```python
from build123d import *

# Parameters (mm, degrees)
F3_DEPTH = 15
F2_R     = 6.1
F4_DEPTH = 20
F5_R     = 3.25
F6_DEPTH = 20
F5_R_2   = 13.7
F7_DEPTH = 1.3
F2_R_2   = 20
F2_R_3   = 8.5
F8_DEPTH = 0.4


with BuildPart() as f1:
    # F0 (on Right) → F1 (revolve)
    with BuildSketch(Plane.YZ):
        with BuildLine():
            Line((0, 10), (0, 0))
            Line((0, 0), (15, 0))
            add(Edge.make_bspline(
                [(12.5, 17.5), (13.5772919142, 11.6888974623), (14.2886459571, 5.8444487312), (15, 0)],
                knots=[0.5019201889, 0.5019201889, 0.5019201889, 0.5019201889, 1, 1, 1, 1], degree=3))
            Line((12.5, 17.5), (8.4409715081, 17.5))
            ThreePointArc((8.4409715081, 17.5), (5.6457948953, 12.1458674864), (0, 10))
        make_face()
        with BuildLine():
            Line((8.4409715081, 17.5), (12.5, 17.5))
            add(Edge.make_bspline(
                [(8.5, 35), (9.9572008854, 29.1779541329), (11.4144017707, 23.3559082658), (12.5, 17.5)],
                knots=[0, 0, 0, 0, 0.5019201889, 0.5019201889, 0.5019201889, 0.5019201889], degree=3))
            Line((8.5, 35), (0, 35))
            Line((0, 35), (0, 27))
            ThreePointArc((0, 27), (6.0104076401, 24.5104076401), (8.5, 18.5))
            ThreePointArc((8.5, 18.5), (8.4852300446, 17.9991296668), (8.4409715081, 17.5))
        make_face()
    revolve(axis=Axis((0, 0, 17.5), (0, 0, -1)))

    # F0 (on Right) → F3 (cut, symmetric)
    with BuildSketch(Plane.YZ):
        with BuildLine():
            Line((0, 17.5), (0, 10))
            ThreePointArc((0, 10), (5.6457948953, 12.1458674864), (8.4409715081, 17.5))
            Line((8.4409715081, 17.5), (0, 17.5))
        make_face()
        with BuildLine():
            ThreePointArc((-8.4409715081, 17.5), (-5.6457948953, 12.1458674864), (0, 10))
            Line((0, 10), (0, 17.5))
            Line((0, 17.5), (-8.4409715081, 17.5))
        make_face()
        with BuildLine():
            ThreePointArc((0, 27), (-6.3541325136, 24.1457948953), (-8.4409715081, 17.5))
            Line((-8.4409715081, 17.5), (0, 17.5))
            Line((0, 17.5), (0, 27))
        make_face()
        with BuildLine():
            Line((0, 27), (0, 17.5))
            Line((0, 17.5), (8.4409715081, 17.5))
            ThreePointArc((8.4409715081, 17.5), (8.4852300446, 17.9991296668), (8.5, 18.5))
            ThreePointArc((8.5, 18.5), (6.0104076401, 24.5104076401), (0, 27))
        make_face()
    extrude(amount=F3_DEPTH, both=True, mode=Mode.SUBTRACT)

    # F2 (on face) → F4 (cut)
    with BuildSketch(Plane.XY.offset(35)):
        Circle(F2_R)
    extrude(amount=-F4_DEPTH, mode=Mode.SUBTRACT)

    # F5 (on face) → F6 (cut)
    with BuildSketch(Plane(origin=(0, 0, 0), x_dir=(1, 0, 0), z_dir=(0, 0, -1))):
        Circle(F5_R)
    extrude(amount=-F6_DEPTH, mode=Mode.SUBTRACT)

    # F5 (on face) → F7 (cut)
    with BuildSketch(Plane(origin=(0, 0, 0), x_dir=(1, 0, 0), z_dir=(0, 0, -1))):
        Circle(F5_R_2)
        Circle(F5_R, mode=Mode.SUBTRACT)
    extrude(amount=-F7_DEPTH, mode=Mode.SUBTRACT)

    # F2 (on face) → F8 (join)
    with BuildSketch(Plane.XY.offset(35)):
        Circle(F2_R_2)
        Circle(F2_R_3, mode=Mode.SUBTRACT)
        Circle(F2_R_3)
        Circle(F2_R, mode=Mode.SUBTRACT)
    extrude(amount=F8_DEPTH)


solid = f1.part
```
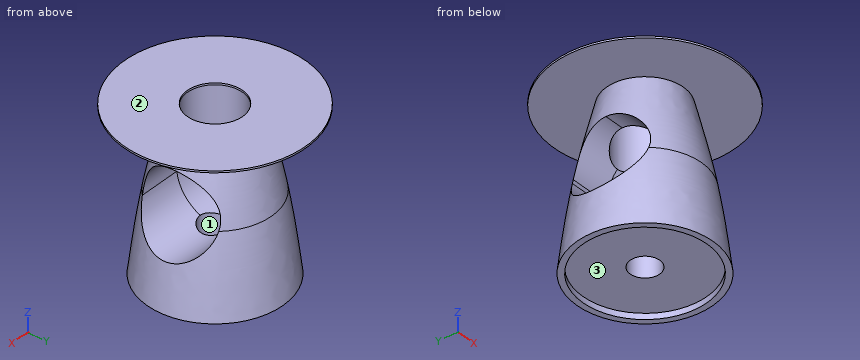
For this review, take the finished solid that the model builds, in its own axes (mm). Face numbers are marked on the shaded views. Round coordinates to 2 decimals unless told otherwise and drop trailing zeros.
Q1. Add section A-A on y = -4.5. Give the number of separate pieces and of enclosed holes in the cut face, plus the area to 3 significant figures.
Result sheet:
separate pieces: 3
enclosed holes: 0
area: 367 mm2
Q2. To check wall thickness, follow line 1 along Z through (x, y) = (1.5, 18); line 2 along Y through (x, z) = (0, 0.5); line 3 along Y through (x, z) = (0, 5). State the ranges of each line that lie inside material, in increasing order.
Result sheet:
line 1: z = 35 to 35.4
line 2: y = -14.94 to -13.7, 13.7 to 14.94
line 3: y = -14.38 to -3.25, 3.25 to 14.38
Q3. Insertion check: pin 1 Ø16 at (x, y) = (0, 0) entering from -Z; pin 2 Ø6 at (y, z) = (10, 14.5) entering from +X; pin 3 Ø4 at (x, z) = (-7, 22) entering from +Y. Each pin has a flat end and moves straight along its axis. Give the tip position at first contact, or say it passes through.
Result sheet:
pin 1: stops at z = 1.3
pin 2: stops at x = 11.07
pin 3: stops at y = 10.57
Q4. Mouldability with a two-part tool opening along X and no side actions: class the marked faces 1, 2 and 3 as +X half, -X half, draft (parallel to the pull), parting line (faces both ways), or undercut.
Result sheet:
face 1: undercut
face 2: draft
face 3: undercut
